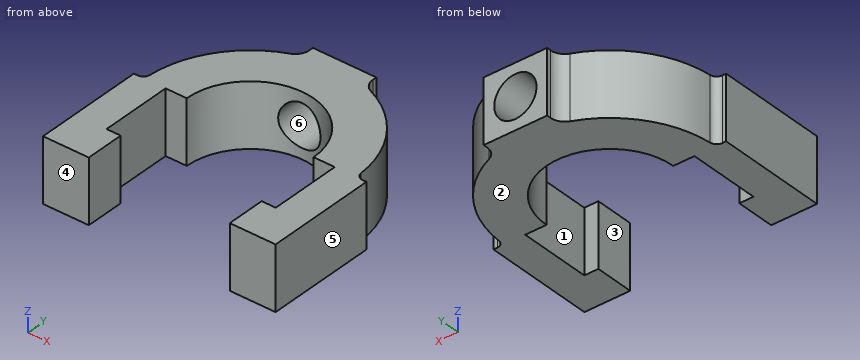
from build123d import *

# Parameters (mm, degrees)
BOSS_EXTRUDE1_DEPTH = 9
FILLET1_R           = 4
FILLET2_R           = 2
HOLE1_D             = 12


with BuildPart() as part:
    # Sketch1 → Boss-Extrude1 (new, symmetric)
    with BuildSketch(Plane.XY):
        with BuildLine():
            Line((-30, 0), (-33, 0))
            Line((-33, 0), (-33, -31.381823957))
            Line((-33, -31.381823957), (-20, -31.381823957))
            Line((-20, -31.381823957), (-20, -20.381823957))
            Line((-20, -20.381823957), (-24, -20.381823957))
            Line((-24, -20.381823957), (-24, 0))
            Line((-24, 0), (-18, 0))
            ThreePointArc((-18, 0), (0, 18), (18, 0))
            Line((18, 0), (24, 0))
            Line((24, 0), (24, -20.381823957))
            Line((24, -20.381823957), (20, -20.381823957))
            Line((20, -20.381823957), (20, -31.381823957))
            Line((20, -31.381823957), (33, -31.381823957))
            Line((33, -31.381823957), (33, 0))
            Line((33, 0), (30, 0))
            ThreePointArc((30, 0), (24.186773245, 17.748239349), (9, 28.618176043))
            Line((9, 28.618176043), (9, 32.618176043))
            Line((9, 32.618176043), (-9, 32.618176043))
            Line((-9, 32.618176043), (-9, 28.618176043))
            ThreePointArc((-9, 28.618176043), (-24.186773245, 17.748239349), (-30, 0))
        make_face()
    extrude(amount=BOSS_EXTRUDE1_DEPTH, both=True)

    # Fillet1
    fillet1_edges = [part.edges().sort_by_distance(p)[0] for p in [
        (-9, 28.618176043, 0),
        (9, 28.618176043, 0),
    ]]
    fillet(fillet1_edges, radius=FILLET1_R)

    # Fillet2
    fillet2_edges = [part.edges().sort_by_distance(p)[0] for p in [
        (30, 0, 0),
        (-30, 0, 0),
    ]]
    fillet(fillet2_edges, radius=FILLET2_R)

    # Hole1 (through all)
    with Locations(Plane(origin=(0, 32.618176043, 0), x_dir=(1, 0, 0), z_dir=(0, 1, 0))):
        with Locations((0, 0)):
            Hole(HOLE1_D / 2)


solid = part.part
The model under review builds one solid part; all positions refer to its coordinate system, in mm. Face numbers are marked on the shaded views. A direction names the side the tool comes from. Coordinates: 2 decimals unless noted, no trailing zeros. Loops run counter-clockwise (first coordinate to the right, second up) from the corner with the lowest first, then second, coordinate; pieces in that order, holes last.
(1) Tool access review of the marked faces 1, 2 and 3: name each direction out of +Z, -Z, +X, -X, +Y, -Y from which nothing blocks a thin tool from reaching the whole face with its end or side.
Determined:
face 1: +Z, -Z
face 2: -Z, +X, -X, +Y, -Y
face 3: +Z, -Z, -Y
(2) Consider section A-A, the plane z = 0. Give the boundary of the cut face in (x, y) (1 decimal).
Determined:
outline: (-33, -31.4) - (-20, -31.4) - (-20, -20.4) - (-24, -20.4) - (-24, 0) - (-18, 0) arc R18 cw to (-6, 17) - (-6, 32.6) - (-9, 32.6) - (-9, 31.4) arc R4 cw to (-11.5, 27.7) arc R30 ccw to (-29.9, 1.9) arc R2 cw to (-31.9, 0) - (-33, 0) - close; (6, 17) arc R18 cw to (18, 0) - (24, 0) - (24, -20.4) - (20, -20.4) - (20, -31.4) - (33, -31.4) - (33, 0) - (31.9, 0) arc R2 cw to (29.9, 1.9) arc R30 ccw to (11.5, 27.7) arc R4 cw to (9, 31.4) - (9, 32.6) - (6, 32.6) - close
(3) Wall thickness on L1, parallel to Z at x = 0, y = 23.25; L2, parallel to X at y = -29, z = 3.5; L3, parallel to X at y = -17, z = 1.25: over which ranges is each line inside the solid? List them lowest first.
Determined:
L1: z = -9 to -6, 6 to 9
L2: x = -33 to -20, 20 to 33
L3: x = -33 to -24, 24 to 33
(4) Consider section B-B, the plane y = -6.5. Give the boundary of the cut face in (x, z), plus the area to 3 significant figures.
Determined:
outline: (-33, -9) - (-24, -9) - (-24, 9) - (-33, 9) - close; (24, -9) - (33, -9) - (33, 9) - (24, 9) - close
area: 324 mm2
(5) Insertion check: P1, Ø6, axis at x = -18, z = -6, coming from the +Y side; P2, Ø0.6, axis at y = 32, z = -2, coming from the +X side; P3, Ø4.5, axis at x = -22.5, z = 0.5, coming from the +Y side; P4, Ø8, axis at x = 17.5, z = 6.5, coming from the -Y side. Each pin has a flat end and moves straight along its axis. Give the tip position at first contact, or say it passes through.
Determined:
P1: stops at y = 25.98
P2: stops at x = 9
P3: stops at y = 22.13
P4: stops at y = -31.38
(6) Draft analysis for pull direction X (two halves, no side actions). For the marked faces 4, 5 and 6, state which applies: +X half, -X half, draft (parallel to the pull), parting line (faces both ways), or undercut.
Determined:
face 4: draft
face 5: +X half
face 6: undercut
(7) Consider section C-C, the plane x = 0. Give the boundary of the cut face in (y, z), plus the area to 3 significant figures.
Determined:
outline: (18, -9) - (32.62, -9) - (32.62, -6) - (18, -6) - close; (18, 6) - (32.62, 6) - (32.62, 9) - (18, 9) - close
area: 87.7 mm2
(8) Consider section D-D, the plane y = 26. Give the boundary of the cut face in (x, z), plus the area to 3 significant figures.
Determined:
outline: (-14.97, -9) - (14.97, -9) - (14.97, 9) - (-14.97, 9) - close; hole circle Ø12 at (0, 0)
area: 426 mm2
